Source: CAD feature listing. Evaluate the final solid. Frame: model axes, mm. Face numbers are marked on the shaded views. Give positions to 0.01 mm unless a question says otherwise; leave off trailing zeros. Write each loop counter-clockwise with the first axis right and the second up, starting at its lowest first coordinate (ties: lowest second). Pieces come first, ordered by that corner, then holes. Notation, with made-up numbers: M 5,10 L 45,10 A15 ccw 45,28 Z; hole C 86,9 d6. An arc over 180 degrees is marked long. Answer as a JSON object with one key per item and string values. Group by question number.
```python
from build123d import *

# Parameters (mm, degrees)
CROQUIS1_R              = 3
SALIENTE_EXTRUIR1_DEPTH = 5
SALIENTE_EXTRUIR2_DEPTH = 16
SALIENTE_EXTRUIR3_DEPTH = 8.2
CROQUIS3_R              = 1.25
CORTAR_EXTRUIR1_DEPTH   = 5


with BuildPart() as part:
    # Croquis1 → Saliente-Extruir1 (new body)
    with BuildSketch(Plane(origin=(0, 308.658769599, 0), x_dir=(1, 0, 0), z_dir=(0, 1, 0))):
        Polygon((-79.783844322, -952.847201319), (-83.742628833, -943.41403856), (-91.093413893, -946.498918444), (-92.641298847, -942.810551303), (-95.774048426, -944.125262056), (-97.550477858, -939.892309261), (-99.87230529, -934.359758549), (-110.937406713, -939.003413413), (-106.839149849, -948.76891692), (-118.762445593, -953.772727382), (-117.214560638, -957.461094523), (-113.313042635, -966.757800174), (-118.964295032, -969.129442753), (-124.496845743, -971.451270185), (-119.85319088, -982.516371608), (-112.357754912, -979.370786552), (-88.272530549, -1036.762099686), (-91.095204728, -1037.946682112), (-96.62775544, -1040.268509543), (-91.984100576, -1051.333610967), (-79.940508545, -1046.279316155), (-75.615152484, -1056.58596144), (-74.067267529, -1060.274328581), (-63.576953324, -1055.871892786), (-59.845268011, -1064.763913767), (-48.780166587, -1060.120258903), (-51.101994019, -1054.587708191), (-52.511851901, -1051.228237922), (-40.595335724, -1046.227272618), (-42.143220678, -1042.538905477), (-46.411310232, -1032.3687173), (-40.753278269, -1029.994229562), (-35.220727557, -1027.67240213), (-39.864382421, -1016.607300707), (-47.366597955, -1019.755730922), (-71.451822317, -962.364417787), (-68.622368572, -961.176990204), (-63.089817861, -958.855162772), (-67.733472724, -947.790061349), align=None)
        with Locations((-88.773377296, -1043.479232823)):
            Circle(CROQUIS1_R, mode=Mode.SUBTRACT)
        with Locations((-56.634544731, -1056.909535623)):
            Circle(CROQUIS1_R, mode=Mode.SUBTRACT)
        with BuildLine():
            Line((-71.509217483, -1036.162059123), (-99.325497684, -967.476035253))
            ThreePointArc((-99.325497684, -967.476035253), (-96.112790855, -959.639858493), (-88.264495604, -962.822846557))
            ThreePointArc((-88.264495604, -962.822846557), (-88.224915609, -962.918213511), (-88.186982587, -963.014247451))
            Line((-88.186982587, -963.014247451), (-71.574392562, -1004.035287893))
            Line((-71.574392562, -1004.035287893), (-65.666191812, -1001.64260073))
            ThreePointArc((-65.666191812, -1001.64260073), (-62.233253946, -1001.525303468), (-59.534729647, -1003.650577014))
            ThreePointArc((-59.534729647, -1003.650577014), (-59.178911441, -1004.342131364), (-58.934639419, -1005.080497936))
            ThreePointArc((-58.934639419, -1005.080497936), (-59.336480357, -1008.551140269), (-61.912548923, -1010.911374385))
            Line((-61.912548923, -1010.911374385), (-67.820749673, -1013.304061547))
            Line((-67.820749673, -1013.304061547), (-60.387770455, -1031.658125581))
            ThreePointArc((-60.387770455, -1031.658125581), (-63.587576477, -1039.516957646), (-71.446408542, -1036.317151624))
            ThreePointArc((-71.446408542, -1036.317151624), (-71.478353691, -1036.239824336), (-71.509217483, -1036.162059123))
        make_face(mode=Mode.SUBTRACT)
        with Locations((-43.075105701, -1024.461678851)):
            Circle(CROQUIS1_R, mode=Mode.SUBTRACT)
        with Locations((-116.6424676, -974.661993465)):
            Circle(CROQUIS1_R, mode=Mode.SUBTRACT)
        with Locations((-103.08302857, -942.214136692)):
            Circle(CROQUIS1_R, mode=Mode.SUBTRACT)
        with Locations((-70.944196004, -955.644439492)):
            Circle(CROQUIS1_R, mode=Mode.SUBTRACT)
    extrude(amount=SALIENTE_EXTRUIR1_DEPTH)

    # Croquis2 → Saliente-Extruir2 (add)
    with BuildSketch(Plane(origin=(0, 313.658769599, 0), x_dir=(1, 0, 0), z_dir=(0, 1, 0))):
        Polygon((-112.357754912, -979.370786552), (-88.272530549, -1036.762099686), (-84.584163408, -1035.214214732), (-108.669387771, -977.822901597), align=None)
        Polygon((-71.451822317, -962.364417787), (-47.366597955, -1019.755730922), (-51.054965096, -1021.303615877), (-75.140189458, -963.912302742), align=None)
        Polygon((-91.093413893, -946.498918444), (-117.214560638, -957.461094523), (-118.762445593, -953.772727382), (-92.641298847, -942.810551303), align=None)
        Polygon((-74.067267529, -1060.274328581), (-63.576953324, -1055.871892786), (-64.157410182, -1054.488755108), (-53.092308759, -1049.845100244), (-52.511851901, -1051.228237922), (-40.595335724, -1046.227272618), (-42.143220678, -1042.538905477), (-75.615152484, -1056.58596144), align=None)
    extrude(amount=SALIENTE_EXTRUIR2_DEPTH)

    # Croquis4 → Saliente-Extruir3 (add)
    with BuildSketch(Plane(origin=(0, 329.658769599, 0), x_dir=(1, 0, 0), z_dir=(0, 1, 0))):
        Polygon((-112.357754912, -979.370786552), (-108.669387771, -977.822901597), (-84.584163408, -1035.214214732), (-88.272530549, -1036.762099686), align=None)
        Polygon((-75.140189458, -963.912302742), (-71.451822317, -962.364417787), (-47.366597955, -1019.755730922), (-51.054965096, -1021.303615877), align=None)
    extrude(amount=SALIENTE_EXTRUIR3_DEPTH)

    # Croquis3 → Cortar-Extruir1 (cut)
    with BuildSketch(Plane(origin=(0, 337.858769599, 0), x_dir=(1, 0, 0), z_dir=(0, 1, 0))):
        with Locations((-101.481612206, -1000.1185865)):
            Circle(CROQUIS3_R)
        with Locations((-107.502918296, -985.770758216)):
            Circle(CROQUIS3_R)
        with Locations((-95.460306115, -1014.466414784)):
            Circle(CROQUIS3_R)
        with Locations((-89.439000024, -1028.814243067)):
            Circle(CROQUIS3_R)
        with Locations((-70.285352842, -970.312274407)):
            Circle(CROQUIS3_R)
        with Locations((-64.264046752, -984.66010269)):
            Circle(CROQUIS3_R)
        with Locations((-52.22143457, -1013.355759258)):
            Circle(CROQUIS3_R)
        with Locations((-58.242740661, -999.007930974)):
            Circle(CROQUIS3_R)
    extrude(amount=-CORTAR_EXTRUIR1_DEPTH, mode=Mode.SUBTRACT)


solid = part.part
```
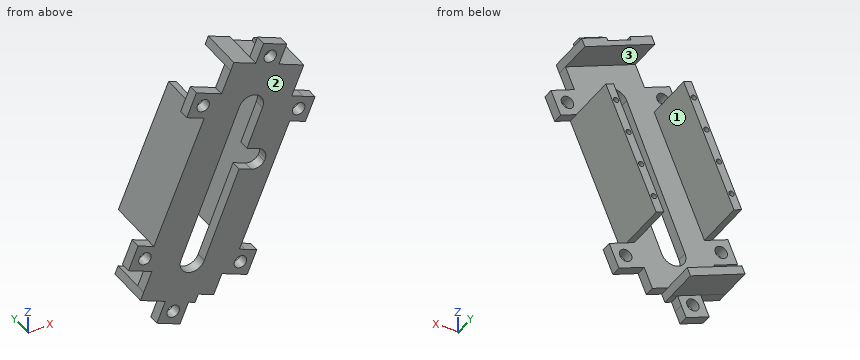
(1) Section D-D, the plane z = 992.5. Return loops of the section in (x, y), plus the area to 3 significant figures.
(2) Section A-A, the plane y = 331. Return loops of the section in (x, z).
(3) Contact query for flat-ended pins moving along their axis: pin 1 Ø10 at (y, z) = (322, 1005.5) entering from -X; pin 2 Ø9.5 at (x, z) = (-116.64, 974.66) entering from +Y; pin 3 Ø0.8 at (x, z) = (-70.5, 970) entering from +Y. Output: stop coordinate, or through.
(4) Section B-B, the plane z = 1007. Return loops of the section in (x, y).
(5) Pull-direction query (X, two-part tool) for the marked faces 1, 2 and 3; classes: pulls with the +X half, pulls with the -X half, needs draft (parallel to the pull), parting line crosses it, or undercut.
(6) Section C-C, the plane y = 321. Return loops of the section in (x, z), plus the area to 3 significant figures.
(7) Ray query, L1, parallel to X at y = 333.5, z = 1000.5; L2, parallel to X at y = 316, z = 1006.5; L3, parallel to X at y = 312.25, z = 976.5. Return the intervals inside material, ascending. Write a range as [from, to].
Reported:
{
 "1": {"outline": "M -106.85,308.66 L -89.19,308.66 L -89.19,313.66 L -102.51,313.66 L -102.51,337.86 L -106.85,337.86 Z; M -76.25,308.66 L -58.8,308.66 L -58.8,337.86 L -63.14,337.86 L -63.14,313.66 L -76.25,313.66 Z", "area": "385 mm2"},
 "2": {"outline": "M -112.36,979.37 L -108.67,977.82 L -84.58,1035.21 L -88.27,1036.76 Z; M -75.14,963.91 L -71.45,962.36 L -47.37,1019.76 L -51.05,1021.3 Z"},
 "3": {"pin 1": "stops at x = -103.49", "pin 2": "stops at y = 313.66", "pin 3": "stops at y = 332.86"},
 "4": {"outline": "M -100.76,308.66 L -83.32,308.66 L -83.32,313.66 L -96.42,313.66 L -96.42,337.86 L -100.76,337.86 Z; M -58.84,308.66 L -52.72,308.66 L -52.72,337.86 L -57.06,337.86 L -57.06,313.66 L -58.84,313.66 Z"},
 "5": {"face 1": "undercut", "face 2": "needs draft", "face 3": "pulls with the -X half"},
 "6": {"outline": "M -118.76,953.77 L -92.64,942.81 L -91.09,946.5 L -117.21,957.46 Z; M -112.36,979.37 L -108.67,977.82 L -84.58,1035.21 L -88.27,1036.76 Z; M -75.62,1056.59 L -42.14,1042.54 L -40.6,1046.23 L -52.51,1051.23 L -53.09,1049.85 L -64.16,1054.49 L -63.58,1055.87 L -74.07,1060.27 Z; M -75.14,963.91 L -71.45,962.36 L -47.37,1019.76 L -51.05,1021.3 Z", "area": "738 mm2"},
 "7": {"L1": "x = [-103.49, -102.67], [-100.29, -99.15], [-59.79, -55.45]", "L2": "x = [-100.97, -96.63], [-57.27, -52.93]", "L3": "x = [-122.38, -119.01], [-114.27, -95.67], [-82.73, -65.52]"}
}
